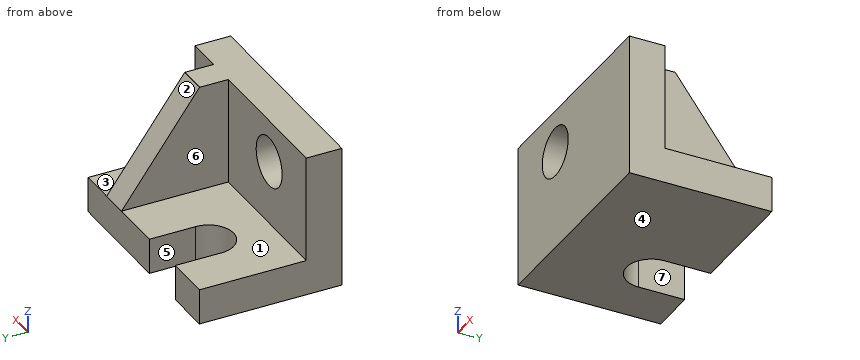
from build123d import *

# Parameters (mm, degrees)
SKETCH_3_W               = 60
SKETCH_3_H               = 40
EXTRUDE_2_DEPTH          = 40
CUT_EXTRUDE_1_DEPTH      = 39
CUT_EXTRUDE_1_DEPTH_BACK = 0.0001
SKETCH_5_W               = 10
SKETCH_5_H               = 30
CUT_EXTRUDE_2_DEPTH      = 43
SKETCH_6_W               = 14
SKETCH_6_H               = 13
CUT_EXTRUDE_3_DEPTH      = 34
SKETCH_7_W               = 14
SKETCH_7_H               = 13
CUT_EXTRUDE_4_DEPTH      = 34
CUT_EXTRUDE_5_DEPTH      = 34
CUT_EXTRUDE_7_DEPTH      = 34
SKETCH_11_R              = 7
CUT_EXTRUDE_8_DEPTH      = 37


with BuildPart() as part:
    # 草图3 → 凸台-拉伸2 (new body)
    with BuildSketch(Plane(origin=(0, 0, 0), x_dir=(1, 0, 0), z_dir=(0, 1, 0))):
        with Locations((-30, -20)):
            Rectangle(SKETCH_3_W, SKETCH_3_H)
    extrude(amount=EXTRUDE_2_DEPTH)

    # 草图4 → 切除-拉伸1 (cut, two sides)
    with BuildSketch(Plane.XY.offset(10)) as cut_extrude_1_sk:
        Polygon((-60, 40), (-47, 40), (-47, 27), (-33, 27), (-33, 40), (-18, 40), (-18, 10), (-60, 10), align=None)
    extrude(amount=CUT_EXTRUDE_1_DEPTH, mode=Mode.SUBTRACT)
    extrude(cut_extrude_1_sk.sketch, amount=-CUT_EXTRUDE_1_DEPTH_BACK, mode=Mode.SUBTRACT)

    # 草图5 → 切除-拉伸2 (cut)
    with BuildSketch(Plane.XY.offset(10)):
        with Locations((-5, 25)):
            Rectangle(SKETCH_5_W, SKETCH_5_H)
    extrude(amount=CUT_EXTRUDE_2_DEPTH, mode=Mode.SUBTRACT)

    # 草图6 → 切除-拉伸3 (cut)
    with BuildSketch(Plane.XY.offset(10)):
        with Locations((-40, 33.5)):
            Rectangle(SKETCH_6_W, SKETCH_6_H)
    extrude(amount=CUT_EXTRUDE_3_DEPTH, mode=Mode.SUBTRACT)

    # 草图7 → 切除-拉伸4 (cut)
    with BuildSketch(Plane.XY.offset(10)):
        with Locations((-40, 33.5)):
            Rectangle(SKETCH_7_W, SKETCH_7_H)
    extrude(amount=-CUT_EXTRUDE_4_DEPTH, mode=Mode.SUBTRACT)

    # 草图8 → 切除-拉伸5 (cut)
    with BuildSketch(Plane.XY.offset(10)):
        with BuildLine():
            Line((-47, 27), (-33, 27))
            ThreePointArc((-33, 27), (-40, 20), (-47, 27))
        make_face()
    extrude(amount=-CUT_EXTRUDE_5_DEPTH, mode=Mode.SUBTRACT)

    # 草图10 → 切除-拉伸7 (cut)
    with BuildSketch(Plane(origin=(0, 0, 0), x_dir=(0, 0, -1), z_dir=(1, 0, 0))):
        Polygon((-40, 40), (-40, 18), (-39.997988347, 18.098350801), (-10, 40), align=None)
    extrude(amount=-CUT_EXTRUDE_7_DEPTH, mode=Mode.SUBTRACT)

    # 草图11 → 切除-拉伸8 (cut)
    with BuildSketch(Plane(origin=(0, 0, 0), x_dir=(1, 0, 0), z_dir=(0, 1, 0))):
        with Locations((-40, -28)):
            Circle(SKETCH_11_R)
    extrude(amount=CUT_EXTRUDE_8_DEPTH, mode=Mode.SUBTRACT)


solid = part.part
Input: part model. Units: mm. Frame: model coordinates. Face numbers are marked on the shaded views. A direction names the side the tool comes from. Give positions to 0.01 mm unless a question says otherwise; leave off trailing zeros. Write each loop counter-clockwise with the first axis right and the second up, starting at its lowest first coordinate (ties: lowest second). Pieces come first, ordered by that corner, then holes. Notation, with made-up numbers: M -3,77 L 35,77 A19 cw 35,101 Z; hole C -22.75,42 d10. An arc over 180 degrees is marked long. Write item = value, one per line. Start each with the question number.
1) Cut plane D-D on y = 17. Return the cut outline in (x, z).
2) First-contact query: pin 1 Ø1.5 at (y, z) = (21, 16.5) entering from -X; pin 2 Ø1.5 at (x, y) = (-17, 31.5) entering from +Z; pin 3 Ø9 at (x, y) = (-39, 23.5) entering from +Z; pin 4 Ø1.5 at (y, z) = (27.5, 30) entering from -X (1 decimal). Flat tips, straight axial feed; report the tip coordinate or a pass-through.
3) Reachability of the marked faces 1, 2 and 3 from +Z, -Z, +X, -X, +Y, -Y: full face, straight path, thin tool, end or side. Return the list, or none.
4) Material intervals for line 1 along X through (y, z) = (6, 28); line 2 along Z through (x, y) = (-40, 6.75); line 3 along Z through (x, y) = (-3.5, 31), sorted ascending. Write a range as [from, to].
5) Cut plane B-B on x = -40. Return the cut outline in (y, z).
6) Cut plane A-A on z = 22. Return the cut outline in (x, y), then the cut area to 3 significant figures.
7) Cut plane C-C on y = 23.5. Return the cut outline in (x, z), then the cut area to 3 significant figures.
8) Draft query along X for the marked faces 4, 5, 6 and 7. Return one class per face: +X half, -X half, draft (parallel to the pull), parting line (faces both ways), or undercut.
Solved:
q1.outline = M -60,0 L 0,0 L 0,10 L -10,10 L -10,40 L -18,40 L -18,10 L -60,10 Z
q2.pin_1 = -18
q2.pin_2 = 22.67
q2.pin_3 = 10
q2.pin_4 = through
q3.face_1 = +Z, -X, +Y
q3.face_2 = +Z, +X, -X, +Y
q3.face_3 = +Z, +X, +Y
q4.line_1 = [-60, -47], [-33, 0]
q4.line_2 = [0, 21], [35, 40]
q4.line_3 = [0, 10]
q5.outline = M 0,0 L 20,0 L 20,10 L 10,10 L 10,21 L 0,21 Z; M 0,35 L 10,35 L 10,40 L 0,40 Z
q6.outline = M -60,0 L -43.61,0 L -43.61,10 L -60,10 Z; M -36.39,0 L 0,0 L 0,10 L -10,10 L -10,31.24 L -18,31.24 L -18,10 L -36.39,10 Z
q6.area = 698 mm2
q7.outline = M -60,0 L -46.06,0 L -46.06,10 L -60,10 Z; M -33.94,0 L 0,0 L 0,10 L -10,10 L -10,32.6 L -18,32.6 L -18,10 L -33.94,10 Z
q7.area = 660 mm2
q8.face_4 = draft
q8.face_5 = undercut
q8.face_6 = -X half
q8.face_7 = undercut
